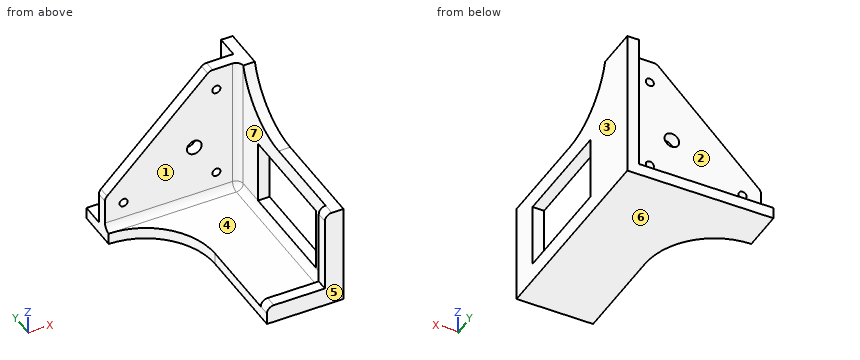
```python
from build123d import *

# Parameters (mm, degrees)
SALIENTE_EXTRUIR1_DEPTH = 5
CROQUIS2_W              = 5
CROQUIS2_H              = 90
SALIENTE_EXTRUIR2_DEPTH = 60
CORTAR_EXTRUIR1_DEPTH   = 5
SALIENTE_EXTRUIR3_DEPTH = 5
REDONDEO1_R             = 3
CROQUIS5_W              = 58
CROQUIS5_H              = 5
SALIENTE_EXTRUIR4_DEPTH = 60
CORTAR_EXTRUIR2_DEPTH   = 5
REDONDEO2_R             = 3
REDONDEO3_R             = 3
CROQUIS7_R              = 1.75
CROQUIS7_R_2            = 3.15
CORTAR_EXTRUIR3_DEPTH   = 5
CROQUIS8_W              = 27.5
CROQUIS8_H              = 47
CORTAR_EXTRUIR4_DEPTH   = 5


with BuildPart() as part:
    # Croquis1 → Saliente-Extruir1 (new body)
    with BuildSketch(Plane.XY):
        with BuildLine():
            Line((-63, 0), (0, 0))
            Line((0, 0), (0, -90))
            Line((0, -90), (-33, -90))
            Line((-33, -90), (-33, -48))
            ThreePointArc((-33, -48), (-41.786797, -26.786797), (-63, -18))
            Line((-63, -18), (-63, 0))
        make_face()
    extrude(amount=SALIENTE_EXTRUIR1_DEPTH)

    # Croquis2 → Saliente-Extruir2 (add)
    with BuildSketch(Plane.XY.offset(5)):
        with Locations((-2.5, -45)):
            Rectangle(CROQUIS2_W, CROQUIS2_H)
    extrude(amount=SALIENTE_EXTRUIR2_DEPTH)

    # Croquis3 → Cortar-Extruir1 (cut)
    with BuildSketch(Plane(origin=(0, 0, 0), x_dir=(0, 0, -1), z_dir=(1, 0, 0))):
        with BuildLine():
            Line((-65, -90), (-43.5, -90))
            Line((-43.5, -90), (-43.5, -46.770645))
            ThreePointArc((-43.5, -46.770645), (-49.46877, -28.81236), (-65, -18))
            Line((-65, -18), (-65, -90))
        make_face()
    extrude(amount=-CORTAR_EXTRUIR1_DEPTH, mode=Mode.SUBTRACT)

    # Croquis4 → Saliente-Extruir3 (add)
    with BuildSketch(Plane.XZ.offset(90)):
        Polygon((-33, 8), (-8, 8), (-8, 43.5), (-5, 43.5), (-5, 5), (-33, 5), align=None)
    extrude(amount=-SALIENTE_EXTRUIR3_DEPTH)

    # Redondeo1
    redondeo1_edges = [part.edges().sort_by_distance(p)[0] for p in [
        (-33, -87.5, 8),
        (-8, -87.5, 43.5),
    ]]
    fillet(redondeo1_edges, radius=REDONDEO1_R)

    # Croquis5 → Saliente-Extruir4 (add)
    with BuildSketch(Plane.XY.offset(5)):
        with Locations((-34, -12.5)):
            Rectangle(CROQUIS5_W, CROQUIS5_H)
    extrude(amount=SALIENTE_EXTRUIR4_DEPTH)

    # Croquis6 → Cortar-Extruir2 (cut)
    with BuildSketch(Plane(origin=(0, -10, 0), x_dir=(1, 0, 0), z_dir=(0, 1, 0))):
        Polygon((-63, -19.817641), (-17.817641, -65), (-63, -65), align=None)
    extrude(amount=-CORTAR_EXTRUIR2_DEPTH, mode=Mode.SUBTRACT)

    # Redondeo2
    redondeo2_edges = [part.edges().sort_by_distance(p)[0] for p in [
        (-63, -12.5, 19.817641),
        (-17.817641, -12.5, 65),
    ]]
    fillet(redondeo2_edges, radius=REDONDEO2_R)

    # Redondeo3
    redondeo3_edges = [part.edges().sort_by_distance(p)[0] for p in [
        (-34, -15, 5),
        (-5, -15, 35),
        (-5, -50, 5),
    ]]
    fillet(redondeo3_edges, radius=REDONDEO3_R)

    # Croquis7 → Cortar-Extruir3 (cut)
    with BuildSketch(Plane(origin=(0, -10, 0), x_dir=(1, 0, 0), z_dir=(0, 1, 0))):
        with Locations((-15, -55)):
            Circle(CROQUIS7_R)
        with Locations((-15, -15)):
            Circle(CROQUIS7_R)
        with Locations((-55, -15)):
            Circle(CROQUIS7_R)
        with Locations((-24.5, -30.5)):
            Circle(CROQUIS7_R_2)
    extrude(amount=-CORTAR_EXTRUIR3_DEPTH, mode=Mode.SUBTRACT)

    # Croquis8 → Cortar-Extruir4 (cut)
    with BuildSketch(Plane(origin=(0, 0, 0), x_dir=(0, 0, -1), z_dir=(1, 0, 0))):
        with Locations((-21.75, -53.5)):
            Rectangle(CROQUIS8_W, CROQUIS8_H)
    extrude(amount=-CORTAR_EXTRUIR4_DEPTH, mode=Mode.SUBTRACT)


solid = part.part
```
Could you check a few things on this model? Use its own coordinates, in mm. Face numbers are marked on the shaded views. A direction names the side the tool comes from. Round coordinates to 2 decimals unless told otherwise and drop trailing zeros. Loops run counter-clockwise (first coordinate to the right, second up) from the corner with the lowest first, then second, coordinate; pieces in that order, holes last. Notation, with made-up numbers: (88.25, -13.75) - (144.25, -13.75) arc R22 cw to (144.25, 6.25) - close; hole circle Ø7 at (72.25, -9). An arc over 180 degrees is marked (long way). Answer in a Markdown table with one row per item. Add a question column.
(1) If we mould it in two halves opening along Y, with no side actions, what happens to the marked faces 4, 5, 6 and 7? For each: pulls with the +Y half, pulls with the -Y half, needs draft (parallel to the pull), parting line crosses it, or undercut.
(2) If we section it at A-A (z = 15): Please give me the cut outline in (x, y).
(3) For the marked faces 1, 2 and 3, which set-ups out of +Z, -Z, +X, -X, +Y, -Y let a thin tool reach every point of the face, with its end or its side?
(4) If we section it at D-D (x = -23.5): Please give me the cut outline in (y, z), plus the area to 3 significant figures.
(5) If we section it at C-C (y = -60.5): Please give me the cut outline in (x, z).
(6) If we section it at B-B (x = -15): Please give me the cut outline in (y, z), plus the area to 3 significant figures.
(7) I'm going to push flat-ended pins straight in: pin 1 (4 mm diameter, centred on x = -23.5, y = -88, fed in from +Z); pin 2 (4 mm diameter, centred on x = -55, z = 15, fed in from +Y); pin 3 (5.5 mm diameter, centred on y = -88, z = 28, fed in from -X); pin 4 (6 mm diameter, centred on x = -37.5, y = -59, fed in from +Z). Where does each tip first touch, or does it pass through?
(8) I need wall thicknesses on line 1 along Z through (x, y) = (-15, -11); line 2 along X through (y, z) = (-11.9, 15); line 3 along Y through (x, z) = (-59.5, 11). Which ranges of each line are inside material? Lowest first, please.
Model answer:
| question | item | result |
|---|---|---|
| 1 | face 4 | undercut |
| 1 | face 5 | pulls with the -Y half |
| 1 | face 6 | needs draft |
| 1 | face 7 | undercut |
| 2 | outline | (-63, -15) - (-56.75, -15) - (-56.75, -10) - (-63, -10) - close; (-53.25, -15) - (-16.75, -15) - (-16.75, -10) - (-53.25, -10) - close; (-13.25, -15) - (-8, -15) arc R3 cw to (-5, -18) - (-5, -30) - (0, -30) - (0, 0) - (-5, 0) - (-5, -10) - (-13.25, -10) - close; (-8, -90) - (0, -90) - (0, -77) - (-5, -77) - (-5, -85) - (-8, -85) - close |
| 3 | face 1 | +Z, -X, -Y |
| 3 | face 2 | +Z, -X, +Y |
| 3 | face 3 | +Z, -Z, +X, +Y, -Y |
| 4 | outline | (-90, 0) - (0, 0) - (0, 5) - (-10, 5) - (-10, 27.51) - (-15, 27.51) - (-15, 8) arc R3 cw to (-18, 5) - (-85, 5) - (-85, 8) - (-90, 8) - close; (-15, 33.49) - (-10, 33.49) - (-10, 59.32) - (-15, 59.32) - close |
| 4 | area | 709 mm² |
| 5 | outline | (-33, 0) - (0, 0) - (0, 8) - (-5, 8) arc R3 cw to (-8, 5) - (-33, 5) - close; (-5, 35.5) - (0, 35.5) - (0, 43.5) - (-5, 43.5) - close |
| 6 | outline | (-90, 0) - (0, 0) - (0, 5) - (-10, 5) - (-10, 13.25) - (-15, 13.25) - (-15, 8) arc R3 cw to (-18, 5) - (-85, 5) - (-85, 8) - (-90, 8) - close; (-15, 16.75) - (-10, 16.75) - (-10, 53.25) - (-15, 53.25) - close; (-15, 56.75) - (-10, 56.75) - (-10, 65) - (-15, 65) - close |
| 6 | area | 732 mm² |
| 7 | pin 1 | stops at z = 8 |
| 7 | pin 2 | stops at y = -10 |
| 7 | pin 3 | stops at x = -8 |
| 7 | pin 4 | passes through |
| 8 | line 1 | z = 0 to 13.25, 16.75 to 53.25, 56.75 to 65 |
| 8 | line 2 | x = -63 to -56.75, -53.25 to -16.75, -13.25 to 0 |
| 8 | line 3 | y = -15 to -10 |
